Read the model definition and answer for the solid it produces. Units are mm, in the model's axes. Face numbers are marked on the shaded views. A direction names the side the tool comes from. Give positions to 0.01 mm unless a question says otherwise; leave off trailing zeros. Order: outer loops, then holes, each group sorted by start corner. A loop starts at its lowest first (then second) coordinate and runs counter-clockwise, first axis right, second up. Notation, with made-up numbers: (-36, -9.5) - (-4, -9.5) arc R8 cw to (-4, 4.5) - close; hole circle Ø4 at (18, -31.75). An arc over 180 degrees is marked (long way). Write item = value, one per line.
Autodesk Inventor part; units mm, degrees
ref_plane "YZ Plane" through (0, 0, 0) normal (1, 0, 0) x (0, 1, 0)
ref_plane "XZ Plane" through (0, 0, 0) normal (0, 1, 0) x (-1, 0, 0)
ref_plane "XY Plane" through (0, 0, 0) normal (0, 0, 1) x (1, 0, 0)
sketch "Sketch_1" plane through (0, 0, 0) normal (0, 0, 1) x (1, 0, 0)
  line L0 (255, 0) -> (-14, 0)
  line L1 (-14, 0) -> (-14, 5.5)
  line L2 (-14, 5.5) -> (-13.5, 6)
  line L3 (-13.5, 6) -> (-0.2, 6)
  arc A0 (-0.2, 6) -> (0, 6.2) centre (-0.2, 6.2) ccw
  line L4 (0, 6.2) -> (0, 7)
  line L5 (0, 7) -> (0.5, 7.5)
  line L6 (0.5, 7.5) -> (240.5, 7.5)
  line L7 (240.5, 7.5) -> (241, 7)
  line L8 (241, 7) -> (241, 6.2)
  arc A1 (241, 6.2) -> (241.2, 6) centre (241.2, 6.2) ccw
  line L9 (241.2, 6) -> (254.5, 6)
  line L10 (254.5, 6) -> (255, 5.5)
  line L11 (255, 5.5) -> (255, 0)
  line L12 (255, 0) -> (-14, 0)
revolve "Revolution1" add sketch "Sketch_1" angle 360 about axis through (255, 0, 0) along (1, 0, 0)
sketch "_____2" plane through (0, 0, 7.5) normal (0, 0, 1) x (1, 0, 0)
  arc A0 (62.5, 2.5) -> (62.5, -2.5) centre (62.5, 0) ccw
  line L0 (62.5, -2.5) -> (77.5, -2.5)
  arc A1 (77.5, -2.5) -> (77.5, 2.5) centre (77.5, 0) ccw
  line L1 (77.5, 2.5) -> (62.5, 2.5)
extrude "Extrusion1" cut sketch "_____2" against normal blind 3
sketch "_____6" plane through (0, 0, 7.5) normal (0, 0, 1) x (1, 0, 0)
  arc A0 (163.5, 2.5) -> (163.5, -2.5) centre (163.5, 0) ccw
  line L0 (163.5, -2.5) -> (178.5, -2.5)
  arc A1 (178.5, -2.5) -> (178.5, 2.5) centre (178.5, 0) ccw
  line L1 (178.5, 2.5) -> (163.5, 2.5)
extrude "Extrusion2" cut sketch "_____6" against normal blind 3
properties part number "NSFRQ15-241-F14-P12-T14-Q12-WKC60-C20-K60-E20_s"
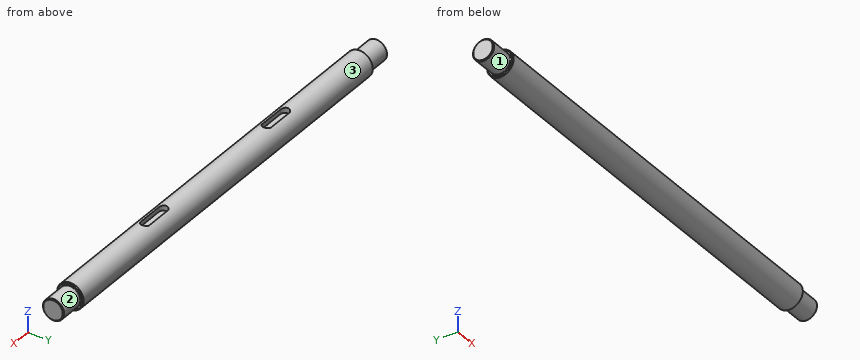
1. For the marked faces 1, 2 and 3, determine the directions among +Z, -Z, +X, -X, +Y, -Y from which every point of the face is accessible in a straight line to the end or side of a thin tool.
Recorded:
face_1 = -X
face_2 = +X
face_3 = +X, -X
2. Straight lines are drawn through the part: L1, parallel to Y at x = 221, z = -0.25; L2, parallel to Y at x = 31.5, z = 2.75; L3, parallel to X at y = -4, z = -5.75. For each, find the intervals that lie inside material, in ascending order. Write a range as [from, to].
Recorded:
L1 = [-7.5, 7.5]
L2 = [-6.98, 6.98]
L3 = [0, 241]
3. Section B-B (x = 216) is taken. Determine the outline of the cut face in (y, z).
Recorded:
outline = circle Ø15 at (0, 0)
4. Flat-ended cylindrical pins translate along their axes: pin 1 (2 mm diameter, centred on x = 67, z = 5.5, fed in from -Y); pin 2 (1.3 mm diameter, centred on x = 69, z = 5.5, fed in from +Y); pin 3 (4 mm diameter, centred on x = 225.5, y = -5.5, fed in from +Z). Find the tip coordinate at first contact, or state that the pin passes through.
Recorded:
pin_1 = -6
pin_2 = 5.72
pin_3 = 6.63
